```python
from build123d import *

# Parameters (mm, degrees)
SKETCH_1_W      = 200
SKETCH_1_H      = 43.4
SKETCH_1_R      = 1.6
EXTRUDE_1_DEPTH = 3


with BuildPart() as part:
    # ｽｹｯﾁ1 → ﾎﾞｽ - 押し出し1 (new body)
    with BuildSketch(Plane.XY):
        Rectangle(SKETCH_1_W, SKETCH_1_H)
        with Locations((-14.557299255, 16.7)):
            Circle(SKETCH_1_R, mode=Mode.SUBTRACT)
        with Locations((-55.557299255, 16.7)):
            Circle(SKETCH_1_R, mode=Mode.SUBTRACT)
        with Locations(Location((14.557299255, 16.7, 0), (0, 0, 180))):
            Circle(SKETCH_1_R, mode=Mode.SUBTRACT)
        with Locations(Location((55.557299255, 16.7, 0), (0, 0, 180))):
            Circle(SKETCH_1_R, mode=Mode.SUBTRACT)
        with Locations((55.557299255, -16.7)):
            Circle(SKETCH_1_R, mode=Mode.SUBTRACT)
        with Locations((14.557299255, -16.7)):
            Circle(SKETCH_1_R, mode=Mode.SUBTRACT)
        with Locations(Location((-55.557299255, -16.7, 0), (0, 0, 180))):
            Circle(SKETCH_1_R, mode=Mode.SUBTRACT)
        with Locations(Location((-14.557299255, -16.7, 0), (0, 0, 180))):
            Circle(SKETCH_1_R, mode=Mode.SUBTRACT)
        with Locations((-95, 8)):
            Circle(SKETCH_1_R, mode=Mode.SUBTRACT)
        with Locations(Location((-95, -8, 0), (0, 0, 180))):
            Circle(SKETCH_1_R, mode=Mode.SUBTRACT)
        with Locations((95, -8)):
            Circle(SKETCH_1_R, mode=Mode.SUBTRACT)
        with Locations(Location((95, 8, 0), (0, 0, 180))):
            Circle(SKETCH_1_R, mode=Mode.SUBTRACT)
    extrude(amount=EXTRUDE_1_DEPTH)


solid = part.part
```
Geometry: final body of the model. Coordinates: model frame, mm. Round coordinates to 2 decimals unless told otherwise and drop trailing zeros. Use one line per item in the form item = value. Start each with the question number.
Q1. Pin query (flat end, axial travel): pin 1 Ø1.9 at (x, y) = (55.56, 16.7) entering from +Z. Return the tip coordinate at first contact, or that it passes through.
Q2. Mould query, pull axis Y, two halves, no side actions, for faces 1 (the face through (55.21, -18.26, 1.48)), 2 (the face through (-93.4, -8.07, 1.48)), 3 (the face through (-1, 0, 3)). Classes: +Y half, -Y half, draft (parallel to the pull), parting line (faces both ways), or undercut.
Q3. Material intervals for line 1 (Y direction, x = -14.5, z = 1.5); line 2 (Y direction, x = -95, z = 1.7); line 3 (X direction, y = -9, z = 1.45), sorted ascending. Write a range as [from, to].
Geometry results:
q1.pin_1 = through
q2.face_1 = undercut
q2.face_2 = undercut
q2.face_3 = draft
q3.line_1 = [-21.7, -18.3], [-15.1, 15.1], [18.3, 21.7]
q3.line_2 = [-21.7, -9.6], [-6.4, 6.4], [9.6, 21.7]
q3.line_3 = [-100, -96.25], [-93.75, 93.75], [96.25, 100]
